Work out the finished part from the listing and answer in its coordinate system (mm). Face numbers are marked on the shaded views. Give positions to 0.01 mm unless a question says otherwise; leave off trailing zeros. Write each loop counter-clockwise with the first axis right and the second up, starting at its lowest first coordinate (ties: lowest second). Pieces come first, ordered by that corner, then holes. Notation, with made-up numbers: (18, 8.25) - (35, 8.25) arc R18 cw to (35, 26.25) - close; hole circle Ø7 at (41.5, 47.25). An arc over 180 degrees is marked (long way). Write item = value, one per line.
Autodesk Inventor part; units mm, degrees
ref_plane "YZ Plane" through (0, 0, 0) normal (1, 0, 0) x (0, 1, 0)
ref_plane "XZ Plane" through (0, 0, 0) normal (0, 1, 0) x (-1, 0, 0)
ref_plane "XY Plane" through (0, 0, 0) normal (0, 0, 1) x (1, 0, 0)
sketch "Sketch1" plane through (0, 0, 0) normal (0, 0, 1) x (1, 0, 0)
  circle A0 centre (0, 0) radius 17.78
  circle A1 centre (0, 0) radius 3.175
  circle A2 centre (0, 0) radius 13.6153
  circle A3 centre (0, 13.6153) radius 1.5875
  circle A4 centre (-11.7912, -6.8077) radius 1.5875
  circle A5 centre (11.7912, -6.8077) radius 1.5875
  dimension "d2" = 27.2307
  dimension "d0" = 35.56
  dimension "d1" = 6.35
  dimension "d3" = 3.175
  dimension "d6" = 360
extrude "Extrusion1" add sketch "Sketch1" along normal blind 12.7 contours A0 | A2 A5 A4 A3
sketch "Sketch2" plane through (0, 0, 12.7) normal (0, 0, 1) x (1, 0, 0)
  point P0 (0, 0)
sketch "Sketch3" plane through (0, 0, 12.7) normal (0, 0, 1) x (1, 0, 0)
  circle A0 centre (0, 13.6153) radius 1.5875
  circle A1 centre (0, 13.6153) radius 3.2766
  circle A2 centre (11.7912, -6.8077) radius 1.5875
  circle A3 centre (11.7912, -6.8077) radius 3.2766
  circle A4 centre (-11.7912, -6.8077) radius 1.5875
  circle A5 centre (-11.7912, -6.8077) radius 3.2766
  point P0 (0, 0)
  dimension "d10" = 6.5532
  dimension "d11" = 6.5532
  dimension "d12" = 6.5532
sketch "Sketch4" plane through (0, 0, 12.7) normal (0, 0, 1) x (1, 0, 0)
  circle A0 centre (0, 0) radius 17.78
  line L0 (-17.78, 0) -> (17.78, 0)
sketch "Sketch5" plane through (0, 0, 12.7) normal (0, 0, 1) x (1, 0, 0)
  circle A0 centre (0, 13.6153) radius 1.5875
  line L0 (0, 13.6153) -> (0, 0)
sketch "Sketch6" plane through (0, 0, 0) normal (0, 1, 0) x (-1, 0, 0)
  point P0 (0, 0)
sketch "Sketch7" plane through (0, 0, 12.7) normal (0, 0, 1) x (1, 0, 0)
  point P0 (0, 0)
properties part number "Burner Table IS v01"
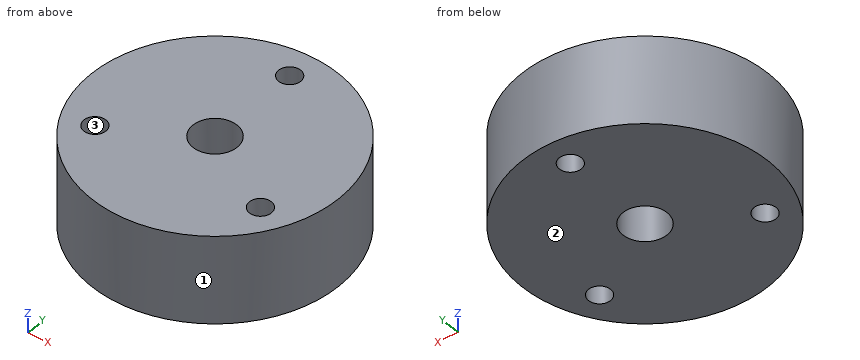
1. Find section A-A, the plane y = 0. Give the vertices of the cut face in (x, z) (3 decimals), then the cut area to 3 significant figures.
Solution:
outline = (-17.78, 0) - (-3.175, 0) - (-3.175, 12.7) - (-17.78, 12.7) - close; (3.175, 0) - (17.78, 0) - (17.78, 12.7) - (3.175, 12.7) - close
area = 371 mm^2
2. Find section B-B, the plane x = 12. Give the vertices of the cut face in (y, z).
Solution:
outline = (-13.12, 0) - (-8.38, 0) - (-8.38, 12.7) - (-13.12, 12.7) - close; (-5.23, 0) - (13.12, 0) - (13.12, 12.7) - (-5.23, 12.7) - close
3. Given pin 1 (4 mm diameter, centred on x = 8.5, z = 8, fed in from -Y); pin 2 (2 mm diameter, centred on x = 1.5, y = 10, fed in from -Z); pin 3 (4 mm diameter, centred on y = 8, z = 3, fed in from -X); pin 4 (3 mm diameter, centred on y = -7.5, z = 11, fed in from +X), each flat-ended and moving along its own axis, determine where each tip first touches the part or whether it passes through.
Solution:
pin_1 = -16.55
pin_2 = 0
pin_3 = -16.74
pin_4 = 16.74
4. Straight lines are drawn through the part: line 1 (Y direction, x = 0, z = 5.75) (3 decimals); line 2 (Y direction, x = 1, z = 10); line 3 (X direction, y = 12.5, z = 2). For each, find the intervals that lie inside material, in ascending order.
Solution:
line_1 = -17.78 to -3.175, 3.175 to 12.028, 15.203 to 17.78
line_2 = -17.75 to -3.01, 3.01 to 12.38, 14.85 to 17.75
line_3 = -12.64 to -1.13, 1.13 to 12.64
5. Find section D-D, the plane x = 6. Give the vertices of the cut face in (y, z).
Solution:
outline = (-16.74, 0) - (16.74, 0) - (16.74, 12.7) - (-16.74, 12.7) - close
6. For a pull along X with two mould halves and no side action, classify the marked faces 1, 2 and 3 as pulls with the +X half, pulls with the -X half, needs draft (parallel to the pull), parting line crosses it, or undercut.
Solution:
face_1 = parting line crosses it
face_2 = needs draft
face_3 = undercut
7. Find section C-C, the plane z = 1. Give the number of separate pieces and of enclosed holes in the cut face, then the cut area to 3 significant figures.
Solution:
separate_pieces = 1
enclosed_holes = 4
area = 938 mm^2
